Autodesk Inventor part; units mm, degrees
ref_plane "Work Plane1" through (3.5, 0, 0) normal (-1, 0, 0) x (0, 0, 1)
ref_plane "YZ Plane" through (0, 0, 0) normal (1, 0, 0) x (0, 1, 0)
ref_plane "XZ Plane" through (0, 0, 0) normal (0, 1, 0) x (-1, 0, 0)
sketch "Sketch1" plane through (0, 0, 0) normal (1, 0, 0) x (0, 1, 0)
  circle A0 centre (0, 0) radius 4
  circle A1 centre (0, 0) radius 11
  dimension "d0" = 8
  dimension "d1" = 22
extrude "Extrusion1" add sketch "Sketch1" along normal blind 7
ref_plane "Work Plane1" through (3.5, 0, 0) normal (-1, 0, 0) x (0, 0, 1)
sketch "Sketch2" plane through (7, 0, 0) normal (1, 0, 0) x (0, 0, -1)
  circle A0 centre (0, 0) radius 4
  circle A1 centre (0, 0) radius 11
  circle A2 centre (0, 0) radius 5
  circle A3 centre (0, 0) radius 10
  dimension "d4" = 1
  dimension "d5" = 1
extrude "Extrusion2" cut sketch "Sketch2" against normal blind 0.5 contours A3
mirror "Mirror1" about plane through (3.5, 0, 0) normal (-1, 0, 0) of "Extrusion2"
properties part number "608bearing"
Source: CAD feature listing. Evaluate the final solid. Frame: model axes, mm. A direction names the side the tool comes from. Give positions to 0.01 mm unless a question says otherwise; leave off trailing zeros. Write each loop counter-clockwise with the first axis right and the second up, starting at its lowest first coordinate (ties: lowest second). Pieces come first, ordered by that corner, then holes. Notation, with made-up numbers: (72, -1) -> (122, -1) arc R19 ccw to (122, 35) -> close; hole circle Ø2 at (71, -16.5). An arc over 180 degrees is marked (long way). Write item = value, one per line.
Q1. First-contact query: pin 1 (2 mm diameter, centred on x = 1.5, y = -2.5, fed in from +Z); pin 2 (1 mm diameter, centred on x = 1, z = -6.5, fed in from -Y); pin 3 (3 mm diameter, centred on y = -7, z = 1.5, fed in from +X); pin 4 (2 mm diameter, centred on y = -1, z = 0.5, fed in from +X). Flat tips, straight axial feed; report the tip coordinate or a pass-through.
Here are the results:
pin_1 = 10.9
pin_2 = -9.22
pin_3 = 6.5
pin_4 = through
Q2. Reachability of faces 1 (the face through (6.75, -4.88, 1.08)), 2 (the face through (3.451, -0.867, 3.905)), 3 (the face through (0.25, 4.88, 1.08)) from +Z, -Z, +X, -X, +Y, -Y: full face, straight path, thin tool, end or side. Return the list, or none.
Here are the results:
face_1 = +X
face_2 = +X, -X
face_3 = -X
Q3. Cut plane C-C on z = 8.25. Return loops of the section in (x, y), then the cut area to 3 significant figures.
Here are the results:
outline = (0, -7.28) -> (7, -7.28) -> (7, -5.65) -> (6.5, -5.65) -> (6.5, 5.65) -> (7, 5.65) -> (7, 7.28) -> (0, 7.28) -> (0, 5.65) -> (0.5, 5.65) -> (0.5, -5.65) -> (0, -5.65) -> close
area = 90.6 mm²
Q4. Mould query, pull axis Z, two halves, no side actions, for faces 4 (the face through (3.45, -2.38, 10.74)), 5 (the face through (0.25, 9.76, 2.17)), 6 (the face through (7, 2, -10)). Classes: +Z half, -Z half, draft (parallel to the pull), parting line (faces both ways), or undercut.
Here are the results:
face_4 = parting line
face_5 = undercut
face_6 = draft
Q5. Cut plane D-D on x = 1. Return loops of the section in (y, z).
Here are the results:
outline = circle Ø22 at (0, 0); hole circle Ø8 at (0, 0)
Q6. Line query: line 1 (X direction, y = -0.75, z = -8); line 2 (Y direction, x = 3, z = -2.25); line 3 (Z direction, x = 3.5, y = 0). Output: solid intervals per line, ascending. Write a range as from..to.
Here are the results:
line_1 = 0.5..6.5
line_2 = -10.77..-3.31, 3.31..10.77
line_3 = -11..-4, 4..11
Q7. Cut plane A-A on y = 0. Return loops of the section in (x, z), then the cut area to 3 significant figures.
Here are the results:
outline = (0, -11) -> (7, -11) -> (7, -10) -> (6.5, -10) -> (6.5, -5) -> (7, -5) -> (7, -4) -> (0, -4) -> (0, -5) -> (0.5, -5) -> (0.5, -10) -> (0, -10) -> close; (0, 4) -> (7, 4) -> (7, 5) -> (6.5, 5) -> (6.5, 10) -> (7, 10) -> (7, 11) -> (0, 11) -> (0, 10) -> (0.5, 10) -> (0.5, 5) -> (0, 5) -> close
area = 88.0 mm²
